CAD build for the part. Positions are in the model's coordinates, mm. A direction names the side the tool comes from. Round coordinates to 2 decimals unless told otherwise and drop trailing zeros. Loops run counter-clockwise (first coordinate to the right, second up) from the corner with the lowest first, then second, coordinate; pieces in that order, holes last. Notation, with made-up numbers: M 36,-8.5 L 46,-8.5 A36 ccw 46,30.5 Z; hole C 62.5,68 d10. An arc over 180 degrees is marked long. Use one line per item in the form item = value.
from build123d import *

# Parameters (mm, degrees)
EXTRUDE_1_DEPTH     = 15
SKETCH_3_R          = 3
CUT_EXTRUDE_1_DEPTH = 15


with BuildPart() as part:
    # 草圖1 → 填料-伸長1 (new body)
    with BuildSketch(Plane(origin=(0, 0, 0), x_dir=(1, 0, 0), z_dir=(0, 1, 0))):
        with BuildLine():
            Line((-200, 55), (-200, -55))
            Line((-200, -55), (-160, -55))
            Line((-160, -55), (-160, -125))
            Line((-160, -125), (-200, -125))
            Line((-200, -125), (-200, -215))
            ThreePointArc((-200, -215), (-197.071067812, -222.071067812), (-190, -225))
            Line((-190, -225), (190, -225))
            ThreePointArc((190, -225), (197.071067812, -222.071067812), (200, -215))
            Line((200, -215), (200, -125))
            Line((200, -125), (160, -125))
            Line((160, -125), (160, -55))
            Line((160, -55), (200, -55))
            Line((200, -55), (200, 55))
            Line((200, 55), (160, 55))
            Line((160, 55), (160, 125))
            Line((160, 125), (200, 125))
            Line((200, 125), (200, 215))
            ThreePointArc((200, 215), (197.071067812, 222.071067812), (190, 225))
            Line((190, 225), (-190, 225))
            ThreePointArc((-190, 225), (-197.071067812, 222.071067812), (-200, 215))
            Line((-200, 215), (-200, 125))
            Line((-200, 125), (-160, 125))
            Line((-160, 125), (-160, 55))
            Line((-160, 55), (-200, 55))
        make_face()
    extrude(amount=EXTRUDE_1_DEPTH)

    # 草圖3 → 除料-伸長1 (cut)
    with BuildSketch(Plane(origin=(0, 15, 0), x_dir=(1, 0, 0), z_dir=(0, 1, 0))):
        with Locations(Location((-130, 125, 0), (0, 0, 270))):
            Circle(SKETCH_3_R)
        with Locations(Location((-100, 125, 0), (0, 0, 270))):
            Circle(SKETCH_3_R)
        with Locations(Location((-100, 55, 0), (0, 0, 90))):
            Circle(SKETCH_3_R)
        with Locations(Location((-130, 55, 0), (0, 0, 90))):
            Circle(SKETCH_3_R)
        with Locations(Location((100, 55, 0), (0, 0, 270))):
            Circle(SKETCH_3_R)
        with Locations(Location((130, 55, 0), (0, 0, 270))):
            Circle(SKETCH_3_R)
        with Locations(Location((100, 125, 0), (0, 0, 90))):
            Circle(SKETCH_3_R)
        with Locations(Location((130, 125, 0), (0, 0, 90))):
            Circle(SKETCH_3_R)
        with Locations(Location((100, -125, 0), (0, 0, 270))):
            Circle(SKETCH_3_R)
        with Locations(Location((130, -125, 0), (0, 0, 270))):
            Circle(SKETCH_3_R)
        with Locations(Location((130, -55, 0), (0, 0, 90))):
            Circle(SKETCH_3_R)
        with Locations(Location((100, -55, 0), (0, 0, 90))):
            Circle(SKETCH_3_R)
        with Locations(Location((-100, -55, 0), (0, 0, 270))):
            Circle(SKETCH_3_R)
        with Locations(Location((-130, -55, 0), (0, 0, 270))):
            Circle(SKETCH_3_R)
        with Locations(Location((-100, -125, 0), (0, 0, 90))):
            Circle(SKETCH_3_R)
        with Locations(Location((-130, -125, 0), (0, 0, 90))):
            Circle(SKETCH_3_R)
        with Locations(Location((-150, -150, 0), (0, 0, 270))):
            Circle(SKETCH_3_R)
        with Locations(Location((150, -150, 0), (0, 0, 270))):
            Circle(SKETCH_3_R)
        with Locations(Location((150, 150, 0), (0, 0, 270))):
            Circle(SKETCH_3_R)
        with Locations(Location((-150, 150, 0), (0, 0, 270))):
            Circle(SKETCH_3_R)
    extrude(amount=-CUT_EXTRUDE_1_DEPTH, mode=Mode.SUBTRACT)


solid = part.part
1. Cut at A-A on x = -168. Write the cut outline in (y, z), and give its area (3 significant figures).
Completed:
outline = M 0,-225 L 15,-225 L 15,-125 L 0,-125 Z; M 0,-55 L 15,-55 L 15,55 L 0,55 Z; M 0,125 L 15,125 L 15,225 L 0,225 Z
area = 4,650 mm2
2. Pull direction Z, two halves, no side cores. Call faces 1 (the face through (200, 7, 171)), 2 (the face through (-196.99, 7.4, -222.15)), 3 (the face through (180, 7, 55)): +Z half, -Z half, draft (parallel to the pull), parting line (faces both ways), or undercut.
Completed:
face_1 = draft
face_2 = -Z half
face_3 = undercut
3. Cut at C-C on z = -109.5. Write the cut outline in (x, y).
Completed:
outline = M -160,0 L 160,0 L 160,15 L -160,15 Z
4. Drop flat-ended pins along their axis: P1, Ø4.5, axis at y = 8.5, z = -83.5, coming from the -X side; P2, Ø6, axis at y = 11, z = -100, coming from the +X side. Give the stop position or say it passes through.
Completed:
P1 = -160
P2 = 160
5. Probe line 1 along Z through (x, y) = (183.5, 6); line 2 along X through (y, z) = (12.5, -126); line 3 along X through (y, z) = (3.75, -148). List the from-to ranges inside material, lowest first. Write a range as from..to.
Completed:
line_1 = -225..-125, -55..55, 125..225
line_2 = -200..-132.83, -127.17..-102.83, -97.17..97.17, 102.83..127.17, 132.83..200
line_3 = -200..-152.24, -147.76..147.76, 152.24..200
6. Cut at B-B on y = 12.5. State how many separate pieces and enclosed holes the cut face has, and give its area (3 significant figures).
Completed:
separate_pieces = 1
enclosed_holes = 20
area = 168,000 mm2
7. Tool access for faces 4 (the face through (-180, 7, -55)), 5 (the face through (196.99, 7.4, 222.15)), 6 (the face through (180, 7, 125)): list every direction of +Z, -Z, +X, -X, +Y, -Y with a clear straight run to the whole face (end or side of a thin tool).
Completed:
face_4 = -X, +Y, -Y
face_5 = +Z, +X, +Y, -Y
face_6 = +X, +Y, -Y
